Can you work these out from the model? Positions are in its coordinate system, mm. A direction names the side the tool comes from. Give positions to 0.01 mm unless a question says otherwise; leave off trailing zeros. Loops run counter-clockwise (first coordinate to the right, second up) from the corner with the lowest first, then second, coordinate; pieces in that order, holes last. Notation, with made-up numbers: M 51,50.25 L 99,50.25 A21 ccw 99,78.25 Z; hole C -30.75,81.5 d5. An arc over 180 degrees is marked long. Answer as a JSON object with one key per item and string values.
```python
from build123d import *

# Parameters (mm, degrees)
F2_R     = 7.9375
F3_DEPTH = 28.576
F4_R     = 5.08


with BuildPart() as f1:
    # F0 (on Right) → F1 (revolve)
    with BuildSketch(Plane.YZ):
        Polygon((28.575, 114.3), (0, 114.3), (0, 73.025), (9.525, 73.025), (9.525, 66.675), (28.575, 66.675), align=None)
    revolve(axis=Axis((0, 0.501314, 0), (0, -1, 0)))

    # F2 (on face) → F3 (cut, through all)
    with BuildSketch(Plane.XZ):
        with Locations((0, 92.075)):
            Circle(F2_R)
        with Locations((-65.106857, 65.106857)):
            Circle(F2_R)
        with Locations((-92.075, 0)):
            Circle(F2_R)
        with Locations((-65.106857, -65.106857)):
            Circle(F2_R)
        with Locations((0, -92.075)):
            Circle(F2_R)
        with Locations((65.106857, -65.106857)):
            Circle(F2_R)
        with Locations((92.075, 0)):
            Circle(F2_R)
        with Locations((65.106857, 65.106857)):
            Circle(F2_R)
    extrude(amount=-F3_DEPTH, mode=Mode.SUBTRACT)

    # F4
    f4_edges = [f1.edges().sort_by_distance(p)[0] for p in [
        (0, 28.575, -114.3),
    ]]
    fillet(f4_edges, radius=F4_R)


solid = f1.part
```
1) Suppose I cut it at A-A, the plane z = 0. Write out the boundary of the cut face in (x, y) (1 decimal), and give its area (3 significant figures).
Answer list:
{"outline": "M -114.3,0 L -100,0 L -100,28.6 L -109.2,28.6 A5.1 ccw -114.3,23.5 Z; M -84.1,0 L -73,0 L -73,9.5 L -66.7,9.5 L -66.7,28.6 L -84.1,28.6 Z; M 66.7,9.5 L 73,9.5 L 73,0 L 84.1,0 L 84.1,28.6 L 66.7,28.6 Z; M 100,0 L 114.3,0 L 114.3,23.5 A5.1 ccw 109.2,28.6 L 100,28.6 Z", "area": "1,680 mm^2"}
2) For faces 4 (the cylindrical face through (99.646, 14.087, 2.384)), 5 (the flat face through (59, 9.525, 32)), which set-ups out of +Z, -Z, +X, -X, +Y, -Y let a thin tool reach every point of the face, with its end or its side?
Answer list:
{"face 4": "+Y, -Y", "face 5": "-Y"}
3) Suppose I cut it at C-C, the plane y = 13.25. Give the number of separate pieces and of enclosed holes in the cut face, and give its area (3 significant figures).
Answer list:
{"separate pieces": "1", "enclosed holes": "9", "area": "25,500 mm^2"}
4) Suppose I cut it at B-B, the plane x = 0. Write out the boundary of the cut face in (y, z) (1 decimal).
Answer list:
{"outline": "M 0,-114.3 L 23.5,-114.3 A5.1 ccw 28.6,-109.2 L 28.6,-100 L 0,-100 Z; M 0,-84.1 L 28.6,-84.1 L 28.6,-66.7 L 9.5,-66.7 L 9.5,-73 L 0,-73 Z; M 0,73 L 9.5,73 L 9.5,66.7 L 28.6,66.7 L 28.6,84.1 L 0,84.1 Z; M 0,100 L 28.6,100 L 28.6,109.2 A5.1 ccw 23.5,114.3 L 0,114.3 Z"}
5) Will these pins go through, and if not, where does the flat tip stop? pin 1 Ø8 at (y, z) = (11, 70) entering from +X; pin 2 Ø1.5 at (y, z) = (3, 9.5) entering from +X; pin 3 Ø1.5 at (x, y) = (-65, 14) entering from +Z; pin 4 Ø10 at (x, z) = (15, 56.5) entering from +Y.
Answer list:
{"pin 1": "x = 93.32", "pin 2": "x = 113.96", "pin 3": "z = 94.53", "pin 4": "through"}
6) If we mould it in two halves opening along Z, with no side actions, what happens to faces 1 (the cylindrical face through (-1.033, 14.087, 99.945)), 2 (the flat face through (-50, 28.575, -47)), 3 (the cylindrical face through (-5.03, 11.58, -114.19))? For each: +Z half, -Z half, draft (parallel to the pull), parting line (faces both ways), or undercut.
Answer list:
{"face 1": "undercut", "face 2": "draft", "face 3": "parting line"}
7) Please list where these lines run through material, in increasing order: line 1 along Z through (x, y) = (0, 16) (1 decimal); line 2 along Z through (x, y) = (0, 6) (1 decimal); line 3 along X through (y, z) = (26.25, -2) (3 decimals). Write a range as from..to.
Answer list:
{"line 1": "-114.3..-100, -84.1..-66.7, 66.7..84.1, 100..114.3", "line 2": "-114.3..-100, -84.1..-73, 73..84.1, 100..114.3", "line 3": "-113.47..-99.756, -84.394..-66.645, 66.645..84.394, 99.756..113.47"}
